from build123d import *

# Parameters (mm, degrees)
SKETCH1_R           = 30
BOSS_EXTRUDE1_DEPTH = 3
SKETCH2_R           = 3.75
BOSS_EXTRUDE2_DEPTH = 10.5
SKETCH3_R           = 4
BOSS_EXTRUDE3_DEPTH = 7.5
BOSS_EXTRUDE4_START = -3
BOSS_EXTRUDE4_DEPTH = 3


with BuildPart() as part:
    # Sketch1 → Boss-Extrude1 (new body)
    with BuildSketch(Plane.XY):
        Circle(SKETCH1_R)
    extrude(amount=BOSS_EXTRUDE1_DEPTH)

    # Sketch2 → Boss-Extrude2 (add)
    with BuildSketch(Plane.XY.offset(3)):
        with Locations(Location((0, 0, 0), (0, 0, 180))):
            Circle(SKETCH2_R)
    extrude(amount=BOSS_EXTRUDE2_DEPTH)

    # Sketch3 → Boss-Extrude3 (add)
    with BuildSketch(Plane.XY.offset(3)):
        with Locations((12, 5)):
            Circle(SKETCH3_R)
    extrude(amount=BOSS_EXTRUDE3_DEPTH)

    # Sketch4 → Boss-Extrude4 (add)
    with BuildSketch(Plane.XY.offset(3).offset(BOSS_EXTRUDE4_START)):
        with BuildLine():
            Line((25.054939633, 16.5), (70, 16.5))
            Line((70, 16.5), (70, -16.5))
            Line((70, -16.5), (25.054939633, -16.5))
            ThreePointArc((25.054939633, -16.5), (30, 0), (25.054939633, 16.5))
        make_face()
    extrude(amount=BOSS_EXTRUDE4_DEPTH)


solid = part.part
Geometry: final body of the model. Coordinates: model frame, mm. A direction names the side the tool comes from. Coordinates: 2 decimals unless noted, no trailing zeros. Order: outer loops, then holes, each group sorted by start corner. A loop starts at its lowest first (then second) coordinate and runs counter-clockwise, first axis right, second up. Notation, with made-up numbers: M -11,43.5 L 3,43.5 A30 cw 3,68.5 Z; hole C 10.25,-2.75 d6. An arc over 180 degrees is marked long. One line per question, with ' | ' between items. Start each with the question number.
Item 1: Cut plane C-C, the plane y = 0. Return the cut outline in (x, z), then the cut area to 3 significant figures.
Item 2: Set-up query: faces 1 (the flat face through (12, 5, 10.5)), 2 (the flat face through (48, -16.5, 1)), 3 (the cylindrical face through (-29.98, 1.07, 1.48)), 4 (the cylindrical face through (-2.02, -3.16, 8.18)). Return all of +Z, -Z, +X, -X, +Y, -Y with unobstructed straight access to the full face (end or side cutting, diameter ignored); none if empty.
Item 3: Pin query (flat end, axial travel): pin 1 Ø3 at (x, y) = (25.5, 9) entering from +Z; pin 2 Ø6 at (x, z) = (13.5, 9) entering from +Y; pin 3 Ø3 at (y, z) = (-8, 2.5) entering from -X; pin 4 Ø1 at (x, z) = (-5, 7) entering from +Y. Return the tip coordinate at first contact, or that it passes through.
Item 4: Cut plane A-A, the plane z = 4.5. Return the cut outline in (x, y).
Item 5: Ray query, probe 1 along Z at (x, y) = (10.5, -25.5); probe 2 along Z at (x, y) = (9, 4); probe 3 along X at (y, z) = (0, 2.5). Return the intervals inside material, ascending. Write a range as [from, to].
Item 6: Cut plane D-D, the plane y = 24. Return the cut outline in (x, z).
Item 7: Draft query along X for faces 5 (the flat face through (70, 0, 1)), 6 (the flat face through (47, 16.5, 1)), 7 (the cylindrical face through (8.8, 2.6, 6.7)). Return one class per face: released by +X, released by -X, zero draft, split by the parting line, or undercut.
Item 8: Cut plane B-B, the plane x = 0. Return the cut outline in (y, z).
A:
1) outline: M -30,0 L 70,0 L 70,3 L 3.75,3 L 3.75,13.5 L -3.75,13.5 L -3.75,3 L -30,3 Z | area: 379 mm2
2) face 1: +Z, +X, +Y, -Y | face 2: +Z, -Z, +X, -Y | face 3: +Z, -Z | face 4: +Z
3) pin 1: stops at z = 3 | pin 2: stops at y = 9 | pin 3: stops at x = -29.29 | pin 4: passes through
4) outline: C 0,0 d7.5; C 12,5 d8
5) probe 1: z = [0, 3] | probe 2: z = [0, 10.5] | probe 3: x = [-30, 70]
6) outline: M -18,0 L 18,0 L 18,3 L -18,3 Z
7) face 5: released by +X | face 6: zero draft | face 7: undercut
8) outline: M -30,0 L 30,0 L 30,3 L 3.75,3 L 3.75,13.5 L -3.75,13.5 L -3.75,3 L -30,3 Z
